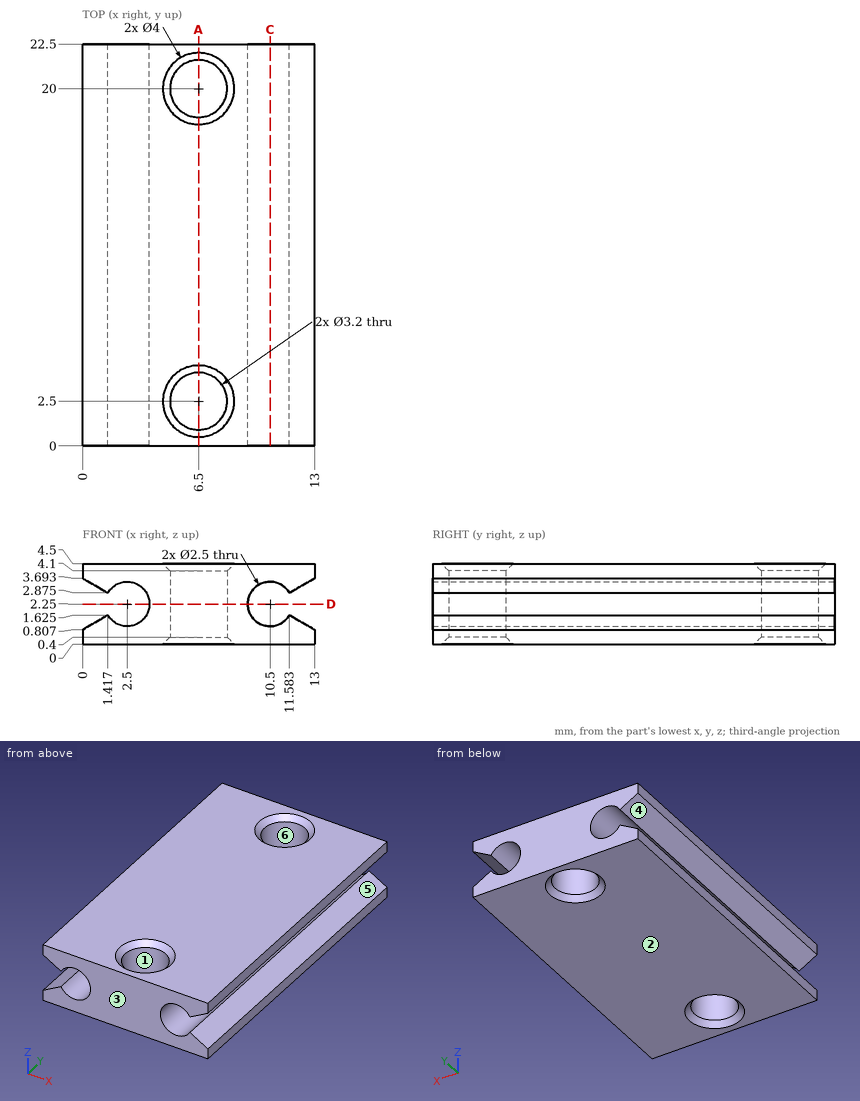
Print and shaded views of the part. All mm, measured from the part's lowest x, y and z. A direction names the side the tool comes from. Coordinates: 2 decimals unless noted, no trailing zeros. Order: outer loops, then holes, each group sorted by start corner. A loop starts at its lowest first (then second) coordinate and runs counter-clockwise, first axis right, second up. Notation, with made-up numbers: (89, 74.25) -> (102, 74.25) arc R9 cw to (102, 78.25) -> close; hole circle Ø9 at (-1, 22). An arc over 180 degrees is marked (long way). Answer as a JSON object with one key per item and string values. Group by question number.
1) Cut at C-C, the plane x = 10.5. Write the cut outline in (y, z).
2) Pull direction Y, two halves, no side cores. Call the marked faces 1, 2 and 3: +Y half, -Y half, draft (parallel to the pull), parting line (faces both ways), or undercut.
3) Flat gauge pins, fed straight in: pin 1 (2.5 mm diameter, centred on x = 6.5, y = 20, fed in from -Z); pin 2 (2 mm diameter, centred on x = 6, z = 1, fed in from -Y); pin 3 (1 mm diameter, centred on y = 12, z = 2, fed in from -X). Where does each tip first touch, or does it go through?
4) Cut at D-D, the plane z = 2.25. Write the cut outline in (x, y).
5) Drill centre lines: L1, parallel to Y at x = 5.5, z = 2.7; L2, parallel to Z at x = 10.5, y = 17; L3, parallel to X at y = 2.25, z = 3.35 (1 decimal). Where is each one in solid material? Low to high.
6) Which spindle directions (+Z, -Z, +X, -X, +Y, -Y) get a long thin tool onto all of the face, cutting with end or side? Do the marked faces 4, 5 and 6. Say none if no direction does.
7) Cut at A-A, the plane x = 6.5. Write the cut outline in (y, z).
Check values:
{
 "1": {"outline": "(0, 0) -> (22.5, 0) -> (22.5, 1) -> (0, 1) -> close; (0, 3.5) -> (22.5, 3.5) -> (22.5, 4.5) -> (0, 4.5) -> close"},
 "2": {"face 1": "undercut", "face 2": "draft", "face 3": "-Y half"},
 "3": {"pin 1": "passes through", "pin 2": "stops at y = 0", "pin 3": "stops at x = 1.2"},
 "4": {"outline": "(3.75, 0) -> (9.25, 0) -> (9.25, 22.5) -> (3.75, 22.5) -> close; hole circle Ø3.2 at (6.5, 2.5); hole circle Ø3.2 at (6.5, 20)"},
 "5": {"L1": "y = 0 to 1.25, 3.75 to 18.75, 21.25 to 22.5", "L2": "z = 0 to 1, 3.5 to 4.5", "L3": "x = 0.6 to 1.9, 3.1 to 4.9, 8.1 to 9.9, 11.1 to 12.4"},
 "6": {"face 4": "-X, +Y, -Y", "face 5": "+X, +Y, -Y", "face 6": "+Z, -Z"},
 "7": {"outline": "(0, 0) -> (0.5, 0) -> (0.9, 0.4) -> (0.9, 4.1) -> (0.5, 4.5) -> (0, 4.5) -> close; (4.1, 0.4) -> (4.5, 0) -> (18, 0) -> (18.4, 0.4) -> (18.4, 4.1) -> (18, 4.5) -> (4.5, 4.5) -> (4.1, 4.1) -> close; (21.6, 0.4) -> (22, 0) -> (22.5, 0) -> (22.5, 4.5) -> (22, 4.5) -> (21.6, 4.1) -> close"}
}
